from build123d import *

# Parameters (mm, degrees)
BOSS_EXTRUDE1_DEPTH = 20
CUT_EXTRUDE1_START  = -4
SKETCH2_R           = 1.625
CUT_EXTRUDE1_DEPTH  = 25
BOSS_EXTRUDE2_DEPTH = 23.4
SKETCH5_R           = 2.75
CUT_EXTRUDE2_DEPTH  = 19
CUT_EXTRUDE3_DEPTH  = 45
CUT_EXTRUDE4_DEPTH  = 20


with BuildPart() as part:
    # Sketch1 → Boss-Extrude1 (new body)
    with BuildSketch(Plane(origin=(0, 0, 0), x_dir=(1, 0, 0), z_dir=(0, 1, 0))):
        Polygon((0, 0), (18.4, 0), (18.4, 20), (31.8, 20), (31.8, 23), (13.4, 23), (13.4, 3), (0, 3), align=None)
    extrude(amount=BOSS_EXTRUDE1_DEPTH)

    # Sketch2 → Cut-Extrude1 (cut)
    with BuildSketch(Plane.XY.offset(-20).offset(CUT_EXTRUDE1_START)):
        with Locations((25.1, 17.5)):
            Circle(SKETCH2_R)
        with Locations((25.1, 2.8)):
            Circle(SKETCH2_R)
    cut_extrude1 = extrude(amount=CUT_EXTRUDE1_DEPTH, mode=Mode.SUBTRACT)

    # Mirror1: Cut-Extrude1 across plane
    add(cut_extrude1.mirror(Plane.ZY.offset(-15.9)), mode=Mode.SUBTRACT)

    # Sketch3 → Boss-Extrude2 (add)
    with BuildSketch(Plane.ZY.offset(-13.4)):
        Polygon((-23, 20), (-23, -24), (-41, -24), (-37, 8), (-37, 20), align=None)
        with BuildLine():
            Line((-28.45, -9), (-28.45, -19))
            ThreePointArc((-28.45, -19), (-31, -21.55), (-33.55, -19))
            Line((-33.55, -19), (-33.55, -9))
            ThreePointArc((-33.55, -9), (-31, -6.45), (-28.45, -9))
        make_face(mode=Mode.SUBTRACT)
    extrude(amount=-BOSS_EXTRUDE2_DEPTH)

    # Sketch5 → Cut-Extrude2 (cut, through all)
    with BuildSketch(Plane.XY.offset(-23)):
        with Locations((25.1, 17.5)):
            Circle(SKETCH5_R)
        with Locations((25.1, 2.8)):
            Circle(SKETCH5_R)
    extrude(amount=-CUT_EXTRUDE2_DEPTH, mode=Mode.SUBTRACT)

    # Sketch4 → Cut-Extrude3 (cut, through all)
    with BuildSketch(Plane.XZ.offset(24)):
        Polygon((36.8, -23), (36.71517637, -41), (36.8, -41), align=None)
    extrude(amount=-CUT_EXTRUDE3_DEPTH, mode=Mode.SUBTRACT)

    # Sketch7 → Cut-Extrude4 (cut)
    with BuildSketch(Plane.ZY.offset(-13.4)):
        with BuildLine():
            Line((-37, -9), (-37, -24))
            Line((-37, -24), (-25, -24))
            Line((-25, -24), (-25, -9))
            ThreePointArc((-25, -9), (-31, -3), (-37, -9))
        make_face()
    extrude(amount=-CUT_EXTRUDE4_DEPTH, mode=Mode.SUBTRACT)


solid = part.part
For this review, take the finished solid that the model builds, in its own axes (mm). A direction names the side the tool comes from. Give positions to 0.01 mm unless a question says otherwise; leave off trailing zeros. Order: outer loops, then holes, each group sorted by start corner. A loop starts at its lowest first (then second) coordinate and runs counter-clockwise, first axis right, second up. Notation, with made-up numbers: (65.25, 77.25) -> (96.25, 77.25) arc R16 ccw to (96.25, 103.25) -> close; hole circle Ø6 at (59.25, 88). An arc over 180 degrees is marked (long way). Write item = value, one per line.
1) We need section A-A, the plane y = 17.5. Give the boundary of the cut face in (x, z) (3 decimals), and give its area (3 significant figures).
Findings:
outline = (0, -3) -> (5.075, -3) -> (5.075, 0) -> (0, 0) -> close; (8.325, -3) -> (13.4, -3) -> (13.4, -37) -> (22.35, -37) -> (22.35, -23) -> (23.475, -23) -> (23.475, -20) -> (18.4, -20) -> (18.4, 0) -> (8.325, 0) -> close; (26.725, -23) -> (27.85, -23) -> (27.85, -37) -> (36.734, -37) -> (36.8, -23) -> (31.8, -23) -> (31.8, -20) -> (26.725, -20) -> close
area = 426 mm^2
2) For faces 1 (the face through (13.4, 8, -22)), 2 (the face through (23, -16, -37)), 3 (the face through (16, 0, -12)), 4 (the face through (24, 16, -23)), list the 3-axis set-ups (+Z, -Z, +X, -X, +Y, -Y) from which the entire face can be reached by the end or side of a thin tool; tool diameter is ignored.
Findings:
face_1 = -Z, -X, +Y, -Y
face_2 = -X, -Y
face_3 = +Z, +X, -X, -Y
face_4 = -Z
3) We need section C-C, the plane z = -31. Give the boundary of the cut face in (x, y).
Findings:
outline = (13.4, -3) -> (33.4, -3) -> (33.4, -6.45) -> (36.76, -6.45) -> (36.76, 20) -> (26.25, 20) arc R2.75 cw (long way) to (23.95, 20) -> (13.4, 20) -> close; (33.4, -24) -> (36.76, -24) -> (36.76, -21.55) -> (33.4, -21.55) -> close; hole circle Ø5.5 at (25.1, 2.8)
4) We need section B-B, the plane x = 6.7. Give the boundary of the cut face in (y, z) (3 decimals).
Findings:
outline = (0, -3) -> (1.175, -3) -> (1.175, 0) -> (0, 0) -> close; (4.425, -3) -> (15.875, -3) -> (15.875, 0) -> (4.425, 0) -> close; (19.125, -3) -> (20, -3) -> (20, 0) -> (19.125, 0) -> close
5) To check wall thickness, follow L1, parallel to X at y = 17.5, z = -21 (3 decimals); L2, parallel to X at y = 17, z = -1; L3, parallel to X at y = 2.5, z = -16.5. State the ranges of each line that lie inside material, in increasing order. Write a range as from..to.
Findings:
L1 = 13.4..23.475, 26.725..31.8
L2 = 0..5.15, 8.25..18.4
L3 = 13.4..18.4
6) Insertion check: pin 1 (6 mm diameter, centred on x = 22, y = 14.5, fed in from -Z); pin 2 (10 mm diameter, centred on y = 9.5, z = -15.5, fed in from +X); pin 3 (10 mm diameter, centred on y = 13, z = -6, fed in from +X). Each pin has a flat end and moves straight along its axis. Give the tip position at first contact, or say it passes through.
Findings:
pin_1 = -37
pin_2 = 31.8
pin_3 = 18.4
7) We need section D-D, the plane x = 14.5. Give the boundary of the cut face in (y, z).
Findings:
outline = (-24, -41) -> (8, -37) -> (20, -37) -> (20, 0) -> (0, 0) -> (0, -23) -> (-24, -23) -> (-24, -25) -> (-9, -25) arc R6 cw to (-9, -37) -> (-24, -37) -> close
8) Draft analysis for pull direction Y (two halves, no side actions). For faces 5 (the face through (35.06, -21.55, -30.94)), 6 (the face through (23, -3, -31)), 7 (the face through (0, 10, -2)), state which applies: pulls with the +Y half, pulls with the -Y half, needs draft (parallel to the pull), parting line crosses it, or undercut.
Findings:
face_5 = undercut
face_6 = pulls with the -Y half
face_7 = needs draft
